Check sheet for the modelled part. Datum: model origin and axes. Units: mm. Coordinates: 2 decimals unless noted, no trailing zeros. Order: outer loops, then holes, each group sorted by start corner. A loop starts at its lowest first (then second) coordinate and runs counter-clockwise, first axis right, second up.
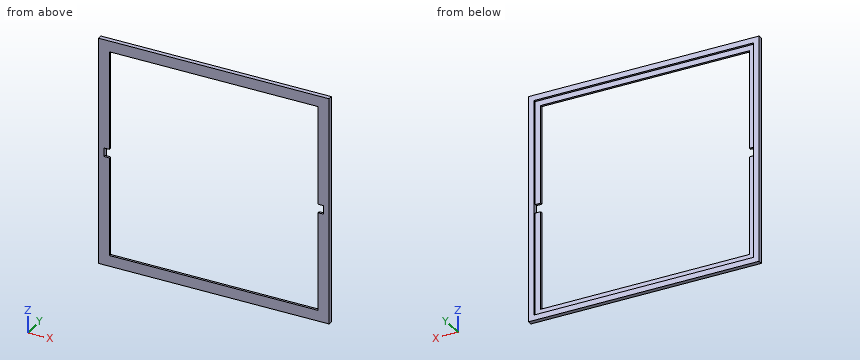
from build123d import *

# Parameters (mm, degrees)
SKETCH1_W           = 210
SKETCH1_H           = 210
SKETCH1_W_2         = 200
SKETCH1_H_2         = 200
BOSS_EXTRUDE1_DEPTH = 2
SKETCH1_4_W         = 210
SKETCH1_4_H         = 210
SKETCH1_4_W_2       = 200
SKETCH1_4_H_2       = 200
BOSS_EXTRUDE2_DEPTH = 4


with BuildPart() as part:
    # Sketch1 → Boss-Extrude1 (new body)
    with BuildSketch(Plane(origin=(0, 0, 0), x_dir=(1, 0, 0), z_dir=(0, 1, 0))):
        with Locations((100, 100)):
            Rectangle(SKETCH1_W, SKETCH1_H)
        with Locations((100, 100)):
            Rectangle(SKETCH1_W_2, SKETCH1_H_2, mode=Mode.SUBTRACT)
        Polygon((0, 96), (0, 0), (200, 0), (200, 96), (195, 96), (195, 5), (5, 5), (5, 96), align=None)
        Polygon((0, 200), (0, 104), (5, 104), (5, 195), (195, 195), (195, 104), (200, 104), (200, 200), align=None)
    extrude(amount=BOSS_EXTRUDE1_DEPTH)

    # Sketch1_4 → Boss-Extrude2 (add)
    with BuildSketch(Plane(origin=(0, 0, 0), x_dir=(1, 0, 0), z_dir=(0, 1, 0))):
        with Locations((100, 100)):
            Rectangle(SKETCH1_4_W, SKETCH1_4_H)
        with Locations((100, 100)):
            Rectangle(SKETCH1_4_W_2, SKETCH1_4_H_2, mode=Mode.SUBTRACT)
    extrude(amount=BOSS_EXTRUDE2_DEPTH)


solid = part.part
(1) Thickness scan on probe 1 along X at (y, z) = (2.3, -16.5); probe 2 along X at (y, z) = (1.3, -17.5); probe 3 along Z at (x, y) = (180, 0.5). Record the ranges inside material, lowest first.
Filled in:
probe 1: x = -5 to 0, 200 to 205
probe 2: x = -5 to 5, 195 to 205
probe 3: z = -205 to -195, -5 to 5
(2) Cross-section at B-B (z = -179). Enter the section's corners in (x, y), and give its area (3 significant figures).
Filled in:
outline: (-5, 0) - (5, 0) - (5, 2) - (0, 2) - (0, 4) - (-5, 4) - close; (195, 0) - (205, 0) - (205, 4) - (200, 4) - (200, 2) - (195, 2) - close
area: 60.0 mm2
(3) Cross-section at C-C (y = 1.35). Enter the section's corners in (x, z).
Filled in:
outline: (-5, -205) - (205, -205) - (205, 5) - (-5, 5) - close; hole (0, -104) - (5, -104) - (5, -195) - (195, -195) - (195, -104) - (200, -104) - (200, -96) - (195, -96) - (195, -5) - (5, -5) - (5, -96) - (0, -96) - close
(4) Cross-section at A-A (x = 59.5). Enter the section's corners in (y, z), and give its area (3 significant figures).
Filled in:
outline: (0, -205) - (4, -205) - (4, -200) - (2, -200) - (2, -195) - (0, -195) - close; (0, -5) - (2, -5) - (2, 0) - (4, 0) - (4, 5) - (0, 5) - close
area: 60.0 mm2
